```python
from build123d import *

# Parameters (mm, degrees)
SKETCH1_W           = 19.05
SKETCH1_H           = 40.64
SKETCH1_H_2         = 6.472052524
BOSS_EXTRUDE1_DEPTH = 3.175
SKETCH1_3_W         = 19.05
SKETCH1_3_H         = 6.472052524
BOSS_EXTRUDE2_DEPTH = 28.575


with BuildPart() as part:
    # Sketch1 → Boss-Extrude1 (new body)
    with BuildSketch(Plane(origin=(0, 0, 0), x_dir=(1, 0, 0), z_dir=(0, 1, 0))):
        Rectangle(SKETCH1_W, SKETCH1_H)
        with Locations((0, 23.556026262)):
            Rectangle(SKETCH1_W, SKETCH1_H_2)
        with Locations((0, -23.556026262)):
            Rectangle(SKETCH1_W, SKETCH1_H_2)
    extrude(amount=BOSS_EXTRUDE1_DEPTH)

    # Sketch1_3 → Boss-Extrude2 (add)
    with BuildSketch(Plane(origin=(0, 0, 0), x_dir=(1, 0, 0), z_dir=(0, 1, 0))):
        with Locations((0, 23.556026262)):
            Rectangle(SKETCH1_3_W, SKETCH1_3_H)
        with Locations((0, -23.556026262)):
            Rectangle(SKETCH1_3_W, SKETCH1_3_H)
    extrude(amount=BOSS_EXTRUDE2_DEPTH)


solid = part.part
```
Part model, mm, in its own coordinate system. A direction names the side the tool comes from. Give positions to 0.01 mm unless a question says otherwise; leave off trailing zeros. Order: outer loops, then holes, each group sorted by start corner. A loop starts at its lowest first (then second) coordinate and runs counter-clockwise, first axis right, second up. Notation, with made-up numbers: M 28,65.5 L 70,65.5 A16 cw 70,85.5 Z; hole C 62,-23.5 d3. An arc over 180 degrees is marked long. Use a Markdown table: item, result. Add a question column.
(1) Probe line 1 along Z through (x, y) = (-5.25, 23); line 2 along Y through (x, z) = (-3, -11) (3 decimals). List the from-to ranges inside material, lowest first. Write a range as [from, to].
(2) Saw through at B-B, the plane x = 8. Give the cut face in (y, z) (3 decimals), and give its area (3 significant figures).
(3) Mould opens along Z. For faces 3 (the face through (0, 14, 26.792)), 4 (the face through (0, 3.175, 0)), 5 (the face through (0, 14, -26.792)) say: +Z half, -Z half, draft (parallel to the pull), parting line (faces both ways), or undercut.
(4) 3-axis set-ups, long thin cutter, end or side, ignore diameter. For faces 1 (the face through (0, 16, -20.32)), 2 (the face through (-9.525, 3, -2)): which of +Z, -Z, +X, -X, +Y, -Y reach the whole face in a straight line?
(5) Saw through at C-C, the plane z = 8. Give the cut face in (x, y) (3 decimals).
(6) Saw through at A-A, the plane y = 8.25. Give the cut face in (x, z) (3 decimals), and give its area (3 significant figures).
(7) Drop a flat-ended pin along its axis: P1, Ø9.5, axis at x = 2.5, z = -0.5, coming from the +Y side (3 decimals). Give the stop position or say it passes through.
Answer key:
| question | item | result |
|---|---|---|
| 1 | line 1 | [-26.79, -20.32], [20.32, 26.79] |
| 1 | line 2 | [0, 3.175] |
| 2 | outline | M 0,-26.792 L 28.575,-26.792 L 28.575,-20.32 L 3.175,-20.32 L 3.175,20.32 L 28.575,20.32 L 28.575,26.792 L 0,26.792 Z |
| 2 | area | 499 mm^2 |
| 3 | face 3 | +Z half |
| 3 | face 4 | undercut |
| 3 | face 5 | -Z half |
| 4 | face 1 | +X, -X, +Y |
| 4 | face 2 | +Z, -Z, -X, +Y, -Y |
| 5 | outline | M -9.525,0 L 9.525,0 L 9.525,3.175 L -9.525,3.175 Z |
| 6 | outline | M -9.525,-26.792 L 9.525,-26.792 L 9.525,-20.32 L -9.525,-20.32 Z; M -9.525,20.32 L 9.525,20.32 L 9.525,26.792 L -9.525,26.792 Z |
| 6 | area | 247 mm^2 |
| 7 | P1 | y = 3.175 |
